The listing builds one solid part. Answer for the finished solid, in the listing's coordinates (mm). Face numbers are marked on the shaded views. A direction names the side the tool comes from. Give positions to 0.01 mm unless a question says otherwise; leave off trailing zeros. Order: outer loops, then holes, each group sorted by start corner. A loop starts at its lowest first (then second) coordinate and runs counter-clockwise, first axis right, second up. Notation, with made-up numbers: M 26.25,63.25 L 44.25,63.25 A6 ccw 44.25,71.25 Z; hole C 43,28 d3. An arc over 180 degrees is marked long. Answer as a JSON object with one key per item and string values. Group by question number.
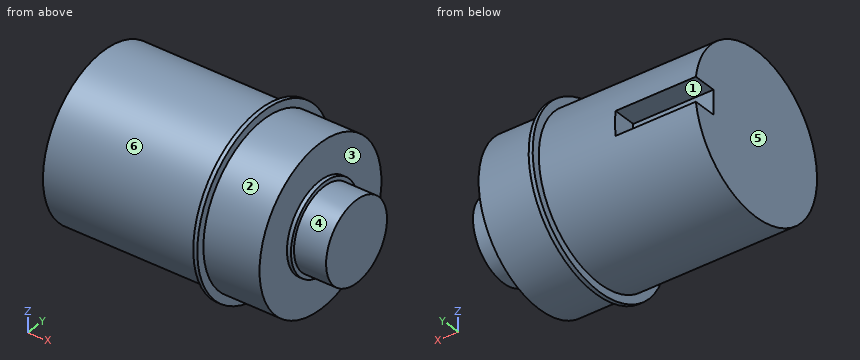
```python
from build123d import *

# Parameters (mm, degrees)
SKETCH1_W          = 0.5
SKETCH1_H          = 1
SKETCH2_W          = 3
SKETCH2_H          = 6
CUT_EXTRUDE1_DEPTH = 10


with BuildPart() as part:
    # Sketch1 → Revolve1 (revolve)
    with BuildSketch(Plane.XY, mode=Mode.PRIVATE) as revolve1_sk:
        Polygon((31.5, 0), (0, 0), (0, 10), (27, 10), (27, 5.5), (27.5, 5.5), (27.5, 5), (31.5, 5), align=None)
        with Locations((19.75, 10.5)):
            Rectangle(SKETCH1_W, SKETCH1_H)
    revolve(revolve1_sk.sketch.rotate(Axis((0, 0, 0), (-1, 0, 0)), 90), axis=Axis((0, 0, 0), (-1, 0, 0)))

    # Sketch2 → Cut-Extrude1 (cut)
    with BuildSketch(Plane.ZY):
        with Locations((0, 10)):
            Rectangle(SKETCH2_W, SKETCH2_H)
    extrude(amount=-CUT_EXTRUDE1_DEPTH, mode=Mode.SUBTRACT)


solid = part.part
```
Item 1: Section B-B (z = 0) is taken. Determine the outline of the cut face in (x, y), and give its area (4 significant figures).
Item 2: A tool of negligible diameter and unlimited length cuts with its end or side. For the marked faces 4, 5 and 6, from which of +Z, -Z, +X, -X, +Y, -Y can it reach the whole face along a straight path? Write none if from no direction.
Item 3: Consider probe 1 along X at (y, z) = (-4.75, 5.5); probe 2 along X at (y, z) = (-9.75, -4.75); probe 3 along Z at (x, y) = (25, 8.75). Determine where each line is inside the solid, lowest interval first. Write a range as from..to.
Item 4: Section D-D (y = -9) is taken. Determine the outline of the cut face in (x, z).
Item 5: Flat-ended cylindrical pins translate along their axes: P1, Ø8, axis at x = 25.5, y = -1.5, coming from the -Z side; P2, Ø0.9, axis at x = 7.5, y = 8.5, coming from the +Z side; P3, Ø1.5, axis at x = 3.5, z = 5.5, coming from the -Y side; P4, Ø6, axis at y = -3.5, z = -4, coming from the +X side. Find the tip coordinate at first contact, or state that the pin passes through.
Item 6: Determine the mould class of the marked faces 1, 2 and 3 for opening direction Z: released by +Z, released by -Z, zero draft, split by the parting line, or undercut.
Item 7: Section C-C (x = 26) is taken. Determine the outline of the cut face in (y, z), and give its area (3 significant figures).
Item 8: Section A-A (y = 0) is taken. Determine the outline of the cut face in (x, z), and give its area (4 significant figures).
Values found:
{
 "1": {"outline": "M 0,-10 L 19.5,-10 L 19.5,-11 L 20,-11 L 20,-10 L 27,-10 L 27,-5.5 L 27.5,-5.5 L 27.5,-5 L 31.5,-5 L 31.5,5 L 27.5,5 L 27.5,5.5 L 27,5.5 L 27,10 L 20,10 L 20,11 L 19.5,11 L 19.5,10 L 10,10 L 10,7 L 0,7 Z", "area": "556.5 mm^2"},
 "2": {"face 4": "+X", "face 5": "+Z, -Z, -X, +Y, -Y", "face 6": "-X"},
 "3": {"probe 1": "x = 0..27", "probe 2": "x = 19.5..20", "probe 3": "z = -4.84..4.84"},
 "4": {"outline": "M 0,-4.36 L 19.5,-4.36 L 19.5,-6.32 L 20,-6.32 L 20,-4.36 L 27,-4.36 L 27,4.36 L 20,4.36 L 20,6.32 L 19.5,6.32 L 19.5,4.36 L 0,4.36 Z"},
 "5": {"P1": "stops at z = -10", "P2": "stops at z = 5.93", "P3": "stops at y = -8.8", "P4": "stops at x = 31.5"},
 "6": {"face 1": "undercut", "face 2": "split by the parting line", "face 3": "zero draft"},
 "7": {"outline": "C 0,0 d20", "area": "314 mm^2"},
 "8": {"outline": "M 0,-10 L 19.5,-10 L 19.5,-11 L 20,-11 L 20,-10 L 27,-10 L 27,-5.5 L 27.5,-5.5 L 27.5,-5 L 31.5,-5 L 31.5,5 L 27.5,5 L 27.5,5.5 L 27,5.5 L 27,10 L 20,10 L 20,11 L 19.5,11 L 19.5,10 L 0,10 Z", "area": "586.5 mm^2"}
}
